Input: part model. Units: mm. Frame: model coordinates. Give positions to 0.01 mm unless a question says otherwise; leave off trailing zeros. Order: outer loops, then holes, each group sorted by start corner. A loop starts at its lowest first (then second) coordinate and runs counter-clockwise, first axis right, second up. Notation, with made-up numbers: (7, -16.5) - (55, -16.5) arc R21 cw to (55, 3.5) - close; hole circle Ø3 at (58.25, 45). An arc over 180 degrees is marked (long way). Answer in a Markdown table with one row per item. Add a question column.
1. Section query D-D on y = 102. Return loops of the section in (x, z).
2. Section query C-C on x = -11. Return loops of the section in (y, z).
3. Section query B-B on z = 3.75. Return loops of the section in (x, y).
4. Contact query for flat-ended pins moving along their axis: pin 1 (1 mm diameter, centred on y = 33, z = 4, fed in from -X); pin 2 (2 mm diameter, centred on y = 47, z = 6.5, fed in from +X); pin 3 (3 mm diameter, centred on y = 100.5, z = 2, fed in from -X). Output: stop coordinate, or through.
5. Ray query, line 1 (X direction, y = 201.5, z = 1); line 2 (Y direction, x = 15, z = 7.25); line 3 (Y direction, x = 24, z = 1.25). Return the intervals inside material, ascending. Write a range as [from, to].
6. Section query A-A on y = 145.5. Return loops of the section in (x, z).
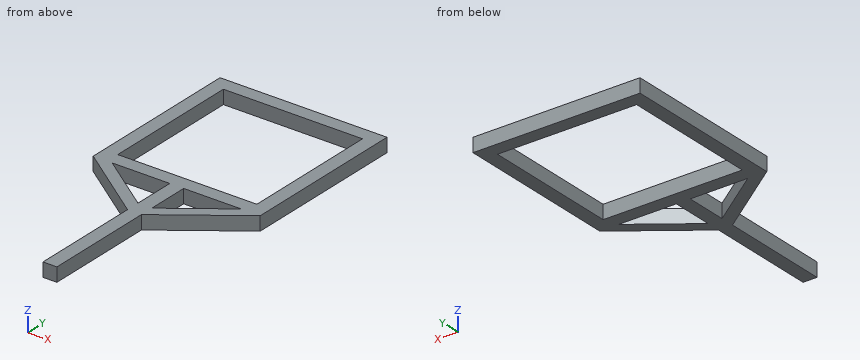
```python
from build123d import *

# Parameters (mm, degrees)
F3_W      = 10
F3_H      = 120
F4_DEPTH  = 10
F7_W      = 120
F7_H      = 10
F8_DEPTH  = 10
F9_W      = 10
F9_H      = 100
F10_DEPTH = 10
F11_W     = 120
F11_H     = 10
F12_DEPTH = 10
F14_DEPTH = 10


with BuildPart() as f4:
    # F3 (on Top) → F4 (new body)
    with BuildSketch(Plane.XY):
        with Locations((0, 60)):
            Rectangle(F3_W, F3_H)
    extrude(amount=F4_DEPTH)

    # F7 (on Top) → F8 (join)
    with BuildSketch(Plane.XY):
        with Locations((0, 125)):
            Rectangle(F7_W, F7_H)
    extrude(amount=F8_DEPTH)

    # F9 (on Top) → F10 (join)
    with BuildSketch(Plane.XY):
        with Locations((-55, 180)):
            Rectangle(F9_W, F9_H)
        with Locations((55, 180)):
            Rectangle(F9_W, F9_H)
    extrude(amount=F10_DEPTH)

    # F11 (on Top) → F12 (join)
    with BuildSketch(Plane.XY):
        with Locations((0, 235)):
            Rectangle(F11_W, F11_H)
    extrude(amount=F12_DEPTH)

    # F13 (on Top) → F14 (join)
    with BuildSketch(Plane.XY):
        Polygon((-5, 80), (-5, 89.891979), (-46.398529, 120), (-60, 120), align=None)
        Polygon((5, 80), (60, 120), (46.398529, 120), (5, 89.891979), align=None)
    extrude(amount=F14_DEPTH)


solid = f4.part
```
Answer:
| question | item | result |
|---|---|---|
| 1 | outline | (-35.25, 0) - (-21.65, 0) - (-21.65, 10) - (-35.25, 10) - close; (-5, 0) - (5, 0) - (5, 10) - (-5, 10) - close; (21.65, 0) - (35.25, 0) - (35.25, 10) - (21.65, 10) - close |
| 2 | outline | (84.36, 0) - (94.26, 0) - (94.26, 10) - (84.36, 10) - close; (120, 0) - (130, 0) - (130, 10) - (120, 10) - close; (230, 0) - (240, 0) - (240, 10) - (230, 10) - close |
| 3 | outline | (-60, 120) - (-5, 80) - (-5, 0) - (5, 0) - (5, 80) - (60, 120) - (60, 240) - (-60, 240) - close; hole (-50, 130) - (50, 130) - (50, 230) - (-50, 230) - close; hole (-46.4, 120) - (-5, 89.89) - (-5, 120) - close; hole (5, 89.89) - (46.4, 120) - (5, 120) - close |
| 4 | pin 1 | stops at x = -5 |
| 4 | pin 2 | stops at x = 5 |
| 4 | pin 3 | stops at x = -35.25 |
| 5 | line 1 | x = [-60, -50], [50, 60] |
| 5 | line 2 | y = [87.27, 97.16], [120, 130], [230, 240] |
| 5 | line 3 | y = [93.82, 103.71], [120, 130], [230, 240] |
| 6 | outline | (-60, 0) - (-50, 0) - (-50, 10) - (-60, 10) - close; (50, 0) - (60, 0) - (60, 10) - (50, 10) - close |
